from build123d import *
from build123d.topology import SkipClean

# Parameters (mm, degrees)
SKETCH_1_R               = 30
EXTRUDE_1_DEPTH          = 8
CUT_EXTRUDE_5_DEPTH      = 905.685953271
CUT_EXTRUDE_5_DEPTH_BACK = 905.685953271
SKETCH_8_R               = 2.25
SKETCH_9_R               = 4
CUT_EXTRUDE_6_DEPTH      = 4.4
FILLET_1_R               = 100
CUT_EXTRUDE_7_DEPTH      = 83
CUT_EXTRUDE_8_DEPTH      = 83
FILLET_3_R               = 100
FILLET_4_R               = 10
SKETCH_14_R              = 4.25
CUT_EXTRUDE_9_DEPTH      = 83
EXTRUDE_2_DEPTH          = 5
FILLET_6_R               = 100
FILLET_7_R               = 10
CHAMFER_1_SIZE           = 5


with BuildPart() as part:
    # 草图1 → 凸台-拉伸1 (new body)
    with BuildSketch(Plane.XY):
        Polygon((0, 250), (769.420884294, 0), (0, 0), (-100, 0), (-869.420884294, 0), (-100, 250), align=None)
        with Locations((50, 100)):
            Circle(SKETCH_1_R, mode=Mode.SUBTRACT)
        with Locations(Location((-150, 100, 0), (0, 0, 180))):
            Circle(SKETCH_1_R, mode=Mode.SUBTRACT)
    extrude(amount=EXTRUDE_1_DEPTH)

    # 草图8 → 切除-拉伸5 (cut, two sides: drawn at the far end of the back side and taken through both)
    with BuildSketch(Plane.XY.offset(8).offset(-CUT_EXTRUDE_5_DEPTH_BACK)):
        with Locations((50, 141.5)):
            Circle(SKETCH_8_R)
        with Locations((79.344931419, 129.344931419)):
            Circle(SKETCH_8_R)
        with Locations((91.5, 100)):
            Circle(SKETCH_8_R)
        with Locations((79.344931419, 70.655068581)):
            Circle(SKETCH_8_R)
        with Locations((50, 58.5)):
            Circle(SKETCH_8_R)
        with Locations((20.655068581, 70.655068581)):
            Circle(SKETCH_8_R)
        with Locations((8.5, 100)):
            Circle(SKETCH_8_R)
        with Locations((20.655068581, 129.344931419)):
            Circle(SKETCH_8_R)
        with Locations(Location((-120.655068581, 129.344931419, 0), (0, 0, 180))):
            Circle(SKETCH_8_R)
        with Locations(Location((-108.5, 100, 0), (0, 0, 180))):
            Circle(SKETCH_8_R)
        with Locations(Location((-120.655068581, 70.655068581, 0), (0, 0, 180))):
            Circle(SKETCH_8_R)
        with Locations(Location((-150, 58.5, 0), (0, 0, 180))):
            Circle(SKETCH_8_R)
        with Locations(Location((-179.344931419, 70.655068581, 0), (0, 0, 180))):
            Circle(SKETCH_8_R)
        with Locations(Location((-191.5, 100, 0), (0, 0, 180))):
            Circle(SKETCH_8_R)
        with Locations(Location((-179.344931419, 129.344931419, 0), (0, 0, 180))):
            Circle(SKETCH_8_R)
        with Locations(Location((-150, 141.5, 0), (0, 0, 180))):
            Circle(SKETCH_8_R)
    extrude(amount=CUT_EXTRUDE_5_DEPTH + CUT_EXTRUDE_5_DEPTH_BACK, mode=Mode.SUBTRACT)

    # 草图9 → 切除-拉伸6 (cut)
    with BuildSketch(Plane.XY.offset(8)):
        with Locations((-150, 141.5)):
            Circle(SKETCH_9_R)
        with Locations((-120.655068581, 129.344931419)):
            Circle(SKETCH_9_R)
        with Locations((-108.5, 100)):
            Circle(SKETCH_9_R)
        with Locations((-120.655068581, 70.655068581)):
            Circle(SKETCH_9_R)
        with Locations((-150, 58.5)):
            Circle(SKETCH_9_R)
        with Locations((-179.344931419, 70.655068581)):
            Circle(SKETCH_9_R)
        with Locations((-191.5, 100)):
            Circle(SKETCH_9_R)
        with Locations((-179.344931419, 129.344931419)):
            Circle(SKETCH_9_R)
        with Locations(Location((79.344931419, 129.344931419, 0), (0, 0, 180))):
            Circle(SKETCH_9_R)
        with Locations(Location((91.5, 100, 0), (0, 0, 180))):
            Circle(SKETCH_9_R)
        with Locations(Location((79.344931419, 70.655068581, 0), (0, 0, 180))):
            Circle(SKETCH_9_R)
        with Locations(Location((50, 58.5, 0), (0, 0, 180))):
            Circle(SKETCH_9_R)
        with Locations(Location((20.655068581, 70.655068581, 0), (0, 0, 180))):
            Circle(SKETCH_9_R)
        with Locations(Location((8.5, 100, 0), (0, 0, 180))):
            Circle(SKETCH_9_R)
        with Locations(Location((20.655068581, 129.344931419, 0), (0, 0, 180))):
            Circle(SKETCH_9_R)
        with Locations(Location((50, 141.5, 0), (0, 0, 180))):
            Circle(SKETCH_9_R)
    extrude(amount=-CUT_EXTRUDE_6_DEPTH, mode=Mode.SUBTRACT)

    # 圆角1
    fillet_1_edges = [part.edges().sort_by_distance(p)[0] for p in [
        (-869.420884294, 0, 4),
        (769.420884294, 0, 4),
    ]]
    fillet(fillet_1_edges, radius=FILLET_1_R)

    # 草图12 → 切除-拉伸7 (cut)
    with BuildSketch(Plane(origin=(0, 0, 0), x_dir=(-1, 0, 0), z_dir=(0, 0, -1))):
        with BuildLine():
            Line((30, 40), (70, 40))
            ThreePointArc((70, 40), (105.27864045, 10.5572809), (150, 0))
            Line((150, 0), (-50, 0))
            ThreePointArc((-50, 0), (-5.27864045, 10.5572809), (30, 40))
        make_face()
    extrude(amount=-CUT_EXTRUDE_7_DEPTH, mode=Mode.SUBTRACT)

    # 草图13 → 切除-拉伸8 (cut)
    with BuildSketch(Plane.XY.offset(8)):
        with BuildLine():
            Line((-238.045732826, 0), (-150, 0))
            ThreePointArc((-150, 0), (-233.430879966, 44.870259677), (-241.990454949, 139.214234639))
            Line((-241.990454949, 139.214234639), (-210, 214.258833414))
            Line((-210, 214.258833414), (-268.947432264, 195.10565163))
            ThreePointArc((-268.947432264, 195.10565163), (-336.814566886, 84.356553496), (-238.045732826, 0))
        make_face()
        with BuildLine():
            Line((110, 214.258833414), (168.947432264, 195.10565163))
            ThreePointArc((168.947432264, 195.10565163), (236.814566886, 84.356553496), (138.045732826, 0))
            Line((138.045732826, 0), (50, 0))
            ThreePointArc((50, 0), (133.430879966, 44.870259677), (141.990454949, 139.214234639))
            Line((141.990454949, 139.214234639), (110, 214.258833414))
        make_face()
    extrude(amount=-CUT_EXTRUDE_8_DEPTH, mode=Mode.SUBTRACT)

    # 圆角3
    fillet_3_edges = [part.edges().sort_by_distance(p)[0] for p in [
        (-100, 250, 4),
        (0, 250, 4),
        (-210, 214.258833414, 4),
        (110, 214.258833414, 4),
    ]]
    fillet(fillet_3_edges, radius=FILLET_3_R)

    # 圆角4
    fillet_4_edges = [part.edges().sort_by_distance(p)[0] for p in [
        (-30, 40, 4),
        (-70, 40, 4),
    ]]
    fillet(fillet_4_edges, radius=FILLET_4_R)

    # 草图14 → 切除-拉伸9 (cut)
    with BuildSketch(Plane.XY.offset(8)):
        with Locations((-35, 65)):
            Circle(SKETCH_14_R)
        with Locations((-35, 105)):
            Circle(SKETCH_14_R)
        with Locations((-35, 175)):
            Circle(SKETCH_14_R)
        with Locations((-35, 215)):
            Circle(SKETCH_14_R)
        with Locations(Location((-65, 215, 0), (0, 0, 180))):
            Circle(SKETCH_14_R)
        with Locations(Location((-65, 175, 0), (0, 0, 180))):
            Circle(SKETCH_14_R)
        with Locations(Location((-65, 105, 0), (0, 0, 180))):
            Circle(SKETCH_14_R)
        with Locations(Location((-65, 65, 0), (0, 0, 180))):
            Circle(SKETCH_14_R)
    extrude(amount=-CUT_EXTRUDE_9_DEPTH, mode=Mode.SUBTRACT)

    # 草图15 → 凸台-拉伸2 (add)
    with SkipClean():  # the faces are left unmerged after this step: merging them gives an invalid solid
        with BuildSketch(Plane(origin=(0, 0, 0), x_dir=(-1, 0, 0), z_dir=(0, 0, -1))):
            with BuildLine():
                Line((-15.063255405, 245.10565163), (-66.7458992, 228.312942707))
                ThreePointArc((-66.7458992, 228.312942707), (-103.346666574, 206.986807031), (-127.834654711, 172.421525717))
                Line((-127.834654711, 172.421525717), (-141.990454949, 139.214234639))
                ThreePointArc((-141.990454949, 139.214234639), (-101.958670135, 14.558226857), (27.138921584, 36.363636364))
                ThreePointArc((27.138921584, 36.363636364), (30.588799415, 39.045340337), (34.852813742, 40))
                Line((34.852813742, 40), (65.147186258, 40))
                ThreePointArc((65.147186258, 40), (69.411200585, 39.045340337), (72.861078416, 36.363636364))
                ThreePointArc((72.861078416, 36.363636364), (201.958670135, 14.558226857), (241.990454949, 139.214234639))
                Line((241.990454949, 139.214234639), (227.834654711, 172.421525717))
                ThreePointArc((227.834654711, 172.421525717), (203.346666574, 206.986807031), (166.7458992, 228.312942707))
                Line((166.7458992, 228.312942707), (115.063255405, 245.10565163))
                ThreePointArc((115.063255405, 245.10565163), (99.805002472, 248.76883406), (84.161555968, 250))
                Line((84.161555968, 250), (15.838444032, 250))
                ThreePointArc((15.838444032, 250), (0.194997528, 248.76883406), (-15.063255405, 245.10565163))
            make_face()
            with BuildLine():
                Line((55, 50), (78.192966918, 50))
                ThreePointArc((78.192966918, 50), (192.379277536, 23.447750944), (230.49164808, 134.312455309))
                Line((230.49164808, 134.312455309), (199.429805152, 207.178675671))
                Line((199.429805152, 207.178675671), (98.416155597, 240))
                Line((98.416155597, 240), (55, 240))
                Line((55, 240), (55, 50))
            make_face(mode=Mode.SUBTRACT)
            with BuildLine():
                Line((45, 240), (45, 50))
                Line((45, 50), (21.807033082, 50))
                ThreePointArc((21.807033082, 50), (-92.379277536, 23.447750944), (-130.49164808, 134.312455309))
                Line((-130.49164808, 134.312455309), (-99.429805152, 207.178675671))
                Line((-99.429805152, 207.178675671), (1.583844403, 240))
                Line((1.583844403, 240), (45, 240))
            make_face(mode=Mode.SUBTRACT)
        extrude(amount=EXTRUDE_2_DEPTH)

    # 圆角6
    fillet_6_edges = [part.edges().sort_by_distance(p)[0] for p in [
        (-199.429805152, 207.178675671, -2.5),
        (99.429805152, 207.178675671, -2.5),
    ]]
    fillet(fillet_6_edges, radius=FILLET_6_R)

    # 圆角7
    fillet_7_edges = [part.edges().sort_by_distance(p)[0] for p in [
        (-98.416155597, 240, -2.5),
        (-55, 240, -2.5),
        (-55, 50, -2.5),
        (-78.192966918, 50, -2.5),
        (-21.807033082, 50, -2.5),
        (-45, 50, -2.5),
        (-45, 240, -2.5),
        (-1.583844403, 240, -2.5),
    ]]
    fillet(fillet_7_edges, radius=FILLET_7_R)

    # 倒角1
    chamfer_1_edges = [part.edges().sort_by_distance(p)[0] for p in [
        (-201.958670135, 14.558226857, 8),
        (-234.91255483, 155.817880178, 8),
        (134.91255483, 155.817880178, 8),
        (-140.904577302, 236.709297168, 8),
        (40.904577302, 236.709297168, 8),
        (-50, 250, 8),
        (-203.346666574, 206.986807031, 8),
        (-99.805002472, 248.76883406, 8),
        (-0.194997528, 248.76883406, 8),
        (103.346666574, 206.986807031, 8),
        (101.958670135, 14.558226857, 8),
        (-50, 40, 8),
        (-30.588799415, 39.045340337, 8),
        (-69.411200585, 39.045340337, 8),
        (-0.194997528, 248.76883406, -5),
        (40.904577302, 236.709297168, -5),
        (103.346666574, 206.986807031, -5),
        (134.91255483, 155.817880178, -5),
        (101.958670135, 14.558226857, -5),
        (-30.588799415, 39.045340337, -5),
        (-50, 40, -5),
        (-69.411200585, 39.045340337, -5),
        (-201.958670135, 14.558226857, -5),
        (-234.91255483, 155.817880178, -5),
        (-203.346666574, 206.986807031, -5),
        (-140.904577302, 236.709297168, -5),
        (-99.805002472, 248.76883406, -5),
        (-50, 250, -5),
    ]]
    chamfer(chamfer_1_edges, length=CHAMFER_1_SIZE - 0.0001)  # a hair under: the kernel refuses the full size


solid = part.part
For this review, take the finished solid that the model builds, in its own axes (mm). A direction names the side the tool comes from. Give positions to 0.01 mm unless a question says otherwise; leave off trailing zeros. Answer in a Markdown table with one row per item. Add a question column.
(1) For pin 1 (6.5 mm diameter, centred on x = -120.66, y = 129.34, fed in from +Z); pin 2 (5.5 mm diameter, centred on y = 138.5, z = -2, fed in from +X); pin 3 (7 mm diameter, centred on x = 20.66, y = 70.66, fed in from -Z), all flat-tipped, find the tip position at first contact; note any pin that passes through.
(2) Mouldability with a two-part tool opening along Y and no side actions: class faces 4 (the face through (-140.505, 234.247, 5.465)), 5 (the face through (-106.654, 96.451, 5.831)) as +Y half, -Y half, draft (parallel to the pull), parting line (faces both ways), or undercut.
(3) Consider section A-A on z = -3. Give the number of separate pieces and of enclosed holes in the cut face, and give its area (3 significant figures).
(4) For faces 1 (the face through (-125, 128, 0)), 2 (the face through (-177.6, 127.6, 3.6)), 3 (the face through (-38.37, 62.41, 4.06)), list the 3-axis set-ups (+Z, -Z, +X, -X, +Y, -Y) from which the entire face can be reached by the end or side of a thin tool; tool diameter is ignored.
(5) Wall thickness on probe 1 along Y at (x, z) = (-150, 6.6); probe 2 along X at (y, z) = (77, -1.5); probe 3 along X at (y, z) = (209.5, -3.5): over which ranges is each line inside the solid? List them lowest first. Write a range as [from, to].
Evaluation:
| question | item | result |
|---|---|---|
| 1 | pin 1 | stops at z = 3.6 |
| 1 | pin 2 | stops at x = 143.06 |
| 1 | pin 3 | stops at z = 0 |
| 2 | face 4 | +Y half |
| 2 | face 5 | undercut |
| 3 | separate pieces | 1 |
| 3 | enclosed holes | 2 |
| 3 | area | 11,200 mm^2 |
| 4 | face 1 | -Z |
| 4 | face 2 | +Z |
| 4 | face 3 | +Z, -Z |
| 5 | probe 1 | y = [3.6, 54.5], [62.5, 70], [130, 137.5], [145.5, 229.97] |
| 5 | probe 2 | x = [-245.78, -234.42], [-55, -45], [134.42, 145.78] |
| 5 | probe 3 | x = [-194.93, -180.49], [-55, -45], [80.49, 94.93] |
